Model file for the job. Use its own axes, mm. A direction names the side the tool comes from. Round coordinates to 2 decimals unless told otherwise and drop trailing zeros. Order: outer loops, then holes, each group sorted by start corner. A loop starts at its lowest first (then second) coordinate and runs counter-clockwise, first axis right, second up. Notation, with made-up numbers: (3.25, 48.5) -> (34.25, 48.5) arc R20 ccw to (34.25, 72.5) -> close; hole circle Ø9 at (27, 26.25). An arc over 180 degrees is marked (long way). Answer as CSV lines item,"result".
```python
from build123d import *

# Parameters (mm, degrees)
SKETCH1_R           = 12.5
BOSS_EXTRUDE1_DEPTH = 50
BOSS_EXTRUDE2_DEPTH = 6
SKETCH3_W           = 6
SKETCH3_H           = 6
CUT_EXTRUDE1_DEPTH  = 119.084715353


with BuildPart() as part:
    # Sketch1 → Boss-Extrude1 (new body)
    with BuildSketch(Plane.XY):
        with BuildLine():
            ThreePointArc((21.164553987, 13.306451613), (20.992319118, 19.401612455), (26.244046944, 22.5))
            Line((26.244046944, 22.5), (50, 22.5))
            Line((50, 22.5), (50, 38))
            Line((50, 38), (-50, 38))
            Line((-50, 38), (-50, 22.5))
            Line((-50, 22.5), (-26.244046944, 22.5))
            ThreePointArc((-26.244046944, 22.5), (-20.992319118, 19.401612455), (-21.164553987, 13.306451613))
            ThreePointArc((-21.164553987, 13.306451613), (-25, 0), (-21.164553987, -13.306451613))
            ThreePointArc((-21.164553987, -13.306451613), (-20.992319118, -19.401612455), (-26.244046944, -22.5))
            Line((-26.244046944, -22.5), (-50, -22.5))
            Line((-50, -22.5), (-50, -38))
            Line((-50, -38), (50, -38))
            Line((50, -38), (50, -22.5))
            Line((50, -22.5), (26.244046944, -22.5))
            ThreePointArc((26.244046944, -22.5), (20.992319118, -19.401612455), (21.164553987, -13.306451613))
            ThreePointArc((21.164553987, -13.306451613), (25, 0), (21.164553987, 13.306451613))
        make_face()
        Circle(SKETCH1_R, mode=Mode.SUBTRACT)
    extrude(amount=BOSS_EXTRUDE1_DEPTH)

    # Sketch2 → Boss-Extrude2 (add)
    with BuildSketch(Plane(origin=(0, 0, 0), x_dir=(-1, 0, 0), z_dir=(0, 0, -1))):
        with BuildLine():
            Line((50, -22.5), (26.244046944, -22.5))
            ThreePointArc((26.244046944, -22.5), (20.992319118, -19.401612455), (21.164553987, -13.306451613))
            ThreePointArc((21.164553987, -13.306451613), (25, 0), (21.164553987, 13.306451613))
            ThreePointArc((21.164553987, 13.306451613), (20.992319118, 19.401612455), (26.244046944, 22.5))
            Line((26.244046944, 22.5), (50, 22.5))
            Line((50, 22.5), (50, -22.5))
        make_face()
        with BuildLine():
            Line((-26.244046944, -22.5), (-50, -22.5))
            Line((-50, -22.5), (-50, 22.5))
            Line((-50, 22.5), (-26.244046944, 22.5))
            ThreePointArc((-26.244046944, 22.5), (-20.992319118, 19.401612455), (-21.164553987, 13.306451613))
            ThreePointArc((-21.164553987, 13.306451613), (-25, 0), (-21.164553987, -13.306451613))
            ThreePointArc((-21.164553987, -13.306451613), (-20.992319118, -19.401612455), (-26.244046944, -22.5))
        make_face()
    extrude(amount=-BOSS_EXTRUDE2_DEPTH)

    # Sketch3 → Cut-Extrude1 (cut, through all)
    with BuildSketch(Plane(origin=(50, 0, 0), x_dir=(0, 0, -1), z_dir=(1, 0, 0))):
        with Locations((-3, 35)):
            Rectangle(SKETCH3_W, SKETCH3_H)
        with Locations((-3, -35)):
            Rectangle(SKETCH3_W, SKETCH3_H)
    extrude(amount=-CUT_EXTRUDE1_DEPTH, mode=Mode.SUBTRACT)


solid = part.part
```
Q1. Saw through at A-A (y = 0). Write the cut outline in (x, z).
Checks:
outline,"(-50, 0) -> (-12.5, 0) -> (-12.5, 50) -> (-25, 50) -> (-25, 6) -> (-50, 6) -> close; (12.5, 0) -> (50, 0) -> (50, 6) -> (25, 6) -> (25, 50) -> (12.5, 50) -> close"
Q2. Wall check: L1, parallel to Y at x = 35, z = 17; L2, parallel to Y at x = 0, z = 28; L3, parallel to Z at x = -25, y = -10.5. Give the ranges that are in metal, low to high. Write a range as [from, to].
Checks:
L1,"[-38, -22.5], [22.5, 38]"
L2,"[-38, -12.5], [12.5, 38]"
L3,"[0, 6]"
Q3. Saw through at D-D (x = -40.5). Write the cut outline in (y, z), plus the area to 3 significant figures.
Checks:
outline,"(-38, 6) -> (-32, 6) -> (-32, 0) -> (32, 0) -> (32, 6) -> (38, 6) -> (38, 50) -> (22.5, 50) -> (22.5, 6) -> (-22.5, 6) -> (-22.5, 50) -> (-38, 50) -> close"
area,"1,750 mm²"
Q4. Saw through at C-C (z = 34). Write the cut outline in (x, y), plus the area to 3 significant figures.
Checks:
outline,"(-50, -38) -> (50, -38) -> (50, -22.5) -> (26.24, -22.5) arc R6 cw to (21.16, -13.31) arc R25 ccw to (21.16, 13.31) arc R6 cw to (26.24, 22.5) -> (50, 22.5) -> (50, 38) -> (-50, 38) -> (-50, 22.5) -> (-26.24, 22.5) arc R6 cw to (-21.16, 13.31) arc R25 ccw to (-21.16, -13.31) arc R6 cw to (-26.24, -22.5) -> (-50, -22.5) -> close; hole circle Ø25 at (0, 0)"
area,"4,650 mm²"
Q5. Flat gauge pins, fed straight in: pin 1 (1.8 mm diameter, centred on x = -16, y = -35.5, fed in from -Z); pin 2 (20 mm diameter, centred on x = 0, y = 0, fed in from -Z); pin 3 (2 mm diameter, centred on y = 5, z = 19, fed in from -X); pin 4 (3 mm diameter, centred on x = 24, z = 3.5, fed in from +Y). Where does each tip first touch, or does it go through?
Checks:
pin 1,"z = 6"
pin 2,"through"
pin 3,"x = -24.68"
pin 4,"y = 32"
Q6. Saw through at B-B (x = 0). Write the cut outline in (y, z).
Checks:
outline,"(-38, 6) -> (-32, 6) -> (-32, 0) -> (-12.5, 0) -> (-12.5, 50) -> (-38, 50) -> close; (12.5, 0) -> (32, 0) -> (32, 6) -> (38, 6) -> (38, 50) -> (12.5, 50) -> close"
Q7. Mould opens along X. For faces 4 (the cylindrical face through (11.923, 3.755, 24.65)), 5 (the flat face through (50, -1, 2)), 6 (the cylindrical face through (-25, 0, 28)), 7 (the flat face through (-1, -38, 28)) say: +X half, -X half, draft (parallel to the pull), parting line (faces both ways), or undercut.
Checks:
face 4,"undercut"
face 5,"+X half"
face 6,"-X half"
face 7,"draft"
Q8. Tool access for faces 1 (the flat face through (1, -35, 6)), 2 (the flat face through (35, 0, 6)), 3 (the flat face through (1, 35, 6)): list every direction of +Z, -Z, +X, -X, +Y, -Y with a clear straight run to the whole face (end or side of a thin tool).
Checks:
face 1,"-Z, +X, -X, -Y"
face 2,"+Z, +X"
face 3,"-Z, +X, -X, +Y"
